Can you work these out from the drawing? Everything is in mm from the part's minimum corner. Round coordinates to 2 decimals unless told otherwise and drop trailing zeros. Loops run counter-clockwise (first coordinate to the right, second up) from the corner with the lowest first, then second, coordinate; pieces in that order, holes last. Notation, with made-up numbers: (38, 83.25) - (92, 83.25) arc R9 ccw to (92, 89.25) - close; hole circle Ø2 at (-39, 25.25). An arc over 180 degrees is marked (long way). Answer as CSV lines item,"result". Start each with the question number.
1) Please list where these lines run through material, in increasing order: line 1 along Y through (x, z) = (7.5, 35); line 2 along Z through (x, y) = (9, 25.25); line 3 along Y through (x, z) = (17.5, 31.5).
2) Suppose I cut it at A-A, the plane z = 35. Write out the boundary of the cut face in (x, y), then the cut area to 3 significant figures.
3) Suppose I cut it at B-B, the plane x = 17.5. Write out the boundary of the cut face in (y, z).
4) We'd pull the mould along X, two halves only. Please class the marked faces 1, 2 and 3: pulls with the +X half, pulls with the -X half, needs draft (parallel to the pull), parting line crosses it, or undercut.
5) Suppose I cut it at C-C, the plane y = 5. Write out the boundary of the cut face in (x, z).
6) Suppose I cut it at D-D, the plane z = 9. Write out the boundary of the cut face in (x, y).
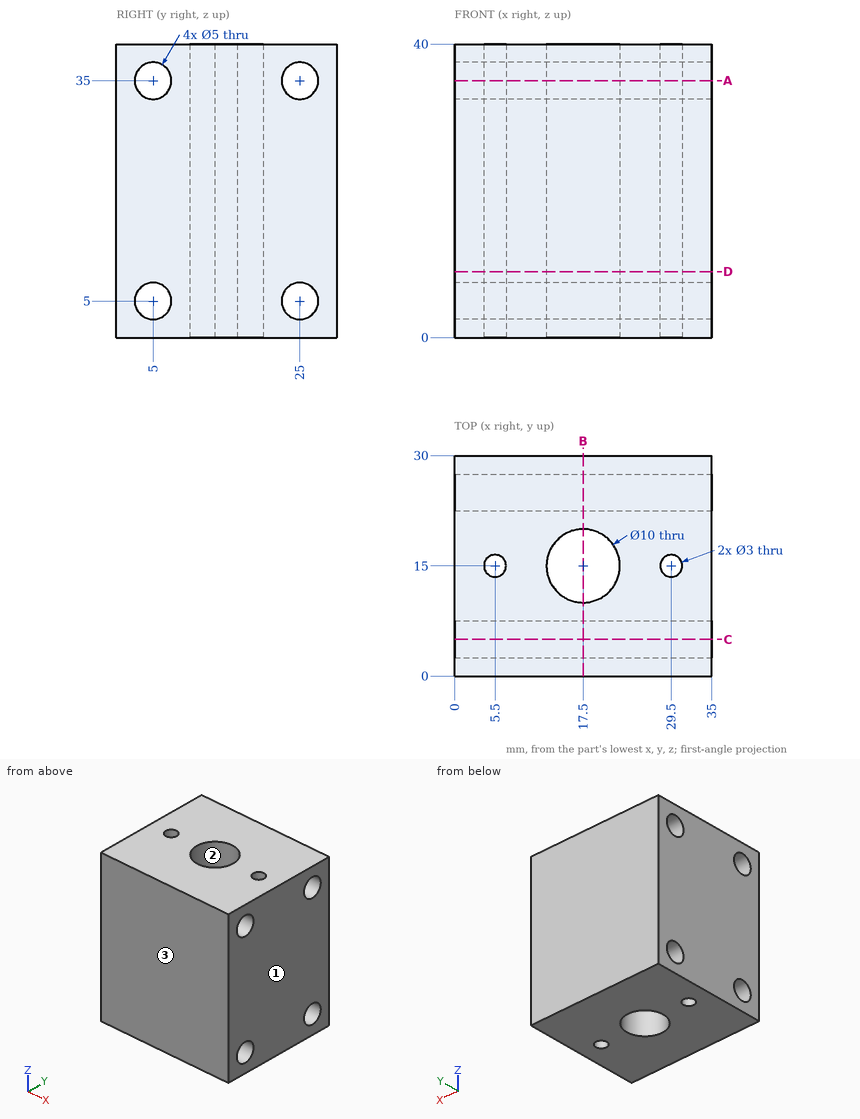
Filled sheet:
1,line 1,"0 to 2.5, 7.5 to 22.5, 27.5 to 30"
1,line 2,"0 to 2.51, 7.49 to 32.51, 37.49 to 40"
1,line 3,"0 to 10, 20 to 30"
2,outline,"(0, 0) - (35, 0) - (35, 2.5) - (0, 2.5) - close; (0, 7.5) - (35, 7.5) - (35, 22.5) - (0, 22.5) - close; (0, 27.5) - (35, 27.5) - (35, 30) - (0, 30) - close; hole circle Ø3 at (5.5, 15); hole circle Ø10 at (17.5, 15); hole circle Ø3 at (29.5, 15)"
2,area,"607 mm²"
3,outline,"(0, 0) - (10, 0) - (10, 40) - (0, 40) - close; (20, 0) - (30, 0) - (30, 40) - (20, 40) - close; hole circle Ø5 at (5, 5); hole circle Ø5 at (5, 35); hole circle Ø5 at (25, 5); hole circle Ø5 at (25, 35)"
4,face 1,"pulls with the +X half"
4,face 2,"undercut"
4,face 3,"needs draft"
5,outline,"(0, 0) - (35, 0) - (35, 2.5) - (0, 2.5) - close; (0, 7.5) - (35, 7.5) - (35, 32.5) - (0, 32.5) - close; (0, 37.5) - (35, 37.5) - (35, 40) - (0, 40) - close"
6,outline,"(0, 0) - (35, 0) - (35, 30) - (0, 30) - close; hole circle Ø3 at (5.5, 15); hole circle Ø10 at (17.5, 15); hole circle Ø3 at (29.5, 15)"
